Autodesk Inventor part; units mm, degrees
ref_plane "bushing_XY" through (0, 4.318, 0) normal (0, -1, 0) x (1, 0, 0)
ref_plane "bushing_YZ" through (0, 4.318, 0) normal (1, 0, 0) x (0, 0, 1)
ref_plane "bushing_ZX" through (0, 4.318, 0) normal (0, 0, 1) x (0, -1, 0)
sketch "Sketch_1" plane through (0, 0, 0) normal (0, 1, 0) x (-1, 0, 0)
  line L0 (3.302, -6.223) -> (3.302, 6.223)
  arc A0 (3.302, 6.223) -> (3.175, 6.35) centre (3.175, 6.223) ccw
  line L1 (3.175, 6.35) -> (-3.175, 6.35)
  arc A1 (-3.175, 6.35) -> (-3.302, 6.223) centre (-3.175, 6.223) ccw
  line L2 (-3.302, 6.223) -> (-3.302, -6.223)
  arc A2 (-3.302, -6.223) -> (-3.175, -6.35) centre (-3.175, -6.223) ccw
  line L3 (-3.175, -6.35) -> (3.175, -6.35)
  arc A3 (3.175, -6.35) -> (3.302, -6.223) centre (3.175, -6.223) ccw
extrude "Extrusion1" add sketch "Sketch_1" along normal mid plane 8.636
sketch "Sketch_2" plane through (3.302, 0, 0) normal (1, 0, 0) x (0, 0, -1)
  line L0 (-3.937, -4.318) -> (-3.683, -4.826)
  line L1 (-3.683, -4.826) -> (-2.667, -4.826)
  line L2 (-2.667, -4.826) -> (-2.413, -4.318)
  line L3 (-2.413, -4.318) -> (-3.937, -4.318)
extrude "Extrusion2" add sketch "Sketch_2" against normal blind 0.635
sketch "Sketch_3" plane through (3.302, 0, 0) normal (1, 0, 0) x (0, 0, -1)
  line L0 (2.413, -4.318) -> (2.667, -4.826)
  line L1 (2.667, -4.826) -> (3.683, -4.826)
  line L2 (3.683, -4.826) -> (3.937, -4.318)
  line L3 (3.937, -4.318) -> (2.413, -4.318)
extrude "Extrusion3" add sketch "Sketch_3" against normal blind 0.635
sketch "Sketch_4" plane through (-3.302, 0, 0) normal (1, 0, 0) x (0, 0, -1)
  line L0 (-3.937, -4.318) -> (-3.683, -4.826)
  line L1 (-3.683, -4.826) -> (-2.667, -4.826)
  line L2 (-2.667, -4.826) -> (-2.413, -4.318)
  line L3 (-2.413, -4.318) -> (-3.937, -4.318)
extrude "Extrusion4" add sketch "Sketch_4" along normal blind 0.635
sketch "Sketch_5" plane through (-3.302, 0, 0) normal (1, 0, 0) x (0, 0, -1)
  line L0 (2.413, -4.318) -> (2.667, -4.826)
  line L1 (2.667, -4.826) -> (3.683, -4.826)
  line L2 (3.683, -4.826) -> (3.937, -4.318)
  line L3 (3.937, -4.318) -> (2.413, -4.318)
extrude "Extrusion5" add sketch "Sketch_5" along normal blind 0.635
ref_plane "bushing_XY" through (0, 4.318, 0) normal (0, -1, 0) x (1, 0, 0)
ref_plane "bushing_YZ" through (0, 4.318, 0) normal (1, 0, 0) x (0, 0, 1)
ref_plane "bushing_ZX" through (0, 4.318, 0) normal (0, 0, 1) x (0, -1, 0)
ref_plane "dummy_body_XY" through (0, 0, 0) normal (0, 1, 0) x (1, 0, 0)
ref_plane "dummy_body_YZ" through (0, 0, 0) normal (1, 0, 0) x (0, 0, -1)
ref_plane "dummy_body_ZX" through (0, 0, 0) normal (0, 0, -1) x (0, 1, 0)
ref_plane "terminals_XY" through (0, -4.191, 0) normal (0, 1, 0) x (1, 0, 0)
ref_plane "terminals_YZ" through (0, -4.191, 0) normal (1, 0, 0) x (0, 0, -1)
ref_plane "terminals_ZX" through (0, -4.191, 0) normal (0, 0, -1) x (0, 1, 0)
properties part number "M2T1S03body"
Source: CAD feature listing. Evaluate the final solid. Frame: model axes, mm. Coordinates: 2 decimals unless noted, no trailing zeros. Loops run counter-clockwise (first coordinate to the right, second up) from the corner with the lowest first, then second, coordinate; pieces in that order, holes last. Notation, with made-up numbers: M 43,-4 L 94,-4 A23 cw 94,6 Z; hole C 18.25,58.5 d10. An arc over 180 degrees is marked long. Put each result on its own line as item: value. Start each with the question number.
1) Cut plane B-B on x = -2.5. Return the cut outline in (y, z), then the cut area to 3 significant figures.
2) Cut plane C-C on z = -4.75. Return the cut outline in (x, y), then the cut area to 3 significant figures.
3) Cut plane A-A on z = -3. Return the cut outline in (x, y), then the cut area to 3 significant figures.
4) Pull-direction query (X, two-part tool) for faces 1 (the face through (0, 4.318, 0)), 2 (the face through (3.302, 0, 0)), 3 (the face through (0, -4.318, 0)); classes: pulls with the +X half, pulls with the -X half, needs draft (parallel to the pull), parting line crosses it, or undercut.
5) Ray query, L1, parallel to Y at x = -2, z = 0.5. Return the intervals inside material, ascending. Write a range as from..to.
The answers:
1. outline: M -4.32,-6.35 L 4.32,-6.35 L 4.32,6.35 L -4.32,6.35 Z
1. area: 110 mm²
2. outline: M -3.3,-4.32 L 3.3,-4.32 L 3.3,4.32 L -3.3,4.32 Z
2. area: 57.0 mm²
3. outline: M -3.3,-4.83 L -2.67,-4.83 L -2.67,-4.32 L 2.67,-4.32 L 2.67,-4.83 L 3.3,-4.83 L 3.3,4.32 L -3.3,4.32 Z
3. area: 57.7 mm²
4. face 1: needs draft
4. face 2: pulls with the +X half
4. face 3: undercut
5. L1: y = -4.32..4.32
